The listing builds one solid part. Answer for the finished solid, in the listing's coordinates (mm). A direction names the side the tool comes from. Coordinates: 2 decimals unless noted, no trailing zeros. Loops run counter-clockwise (first coordinate to the right, second up) from the corner with the lowest first, then second, coordinate; pieces in that order, holes last. Notation, with made-up numbers: (38.5, 38.25) - (87.5, 38.25) arc R24 cw to (87.5, 50.25) - close; hole circle Ø6 at (7, 65.25). An arc over 180 degrees is marked (long way). Use one line per item in the form item = value. Start each with the question number.
Autodesk Inventor part; units mm, degrees
ref_plane "YZ Plane" through (0, 0, 0) normal (1, 0, 0) x (0, 1, 0)
ref_plane "XZ Plane" through (0, 0, 0) normal (0, 1, 0) x (-1, 0, 0)
ref_plane "XY Plane" through (0, 0, 0) normal (0, 0, 1) x (1, 0, 0)
sketch "スケッチ1" plane through (0, 0, 0) normal (0, 1, 0) x (-1, 0, 0)
  line L0 (22.5, -27.3) -> (-22.5, -27.3)
  line L1 (-22.5, -27.3) -> (-22.5, 27.3)
  line L2 (-22.5, 27.3) -> (22.5, 27.3)
  line L3 (22.5, 27.3) -> (22.5, -27.3)
  line L4 (22.5, -27.3) -> (-22.5, 27.3) construction
  line L5 (-22.5, -27.3) -> (22.5, 27.3) construction
  point P0 (0, 0)
  dimension "d0" = 45
  dimension "d1" = 54.6
extrude "押し出し1" add sketch "スケッチ1" along normal blind 5
sketch "スケッチ2" plane through (0, 5, 0) normal (0, 1, 0) x (1, 0, 0)
  line L0 (-22.5, 27.3) -> (-22.5, -27.3)
  line L1 (-22.5, -27.3) -> (22.5, -27.3)
  line L2 (22.5, 27.3) -> (-22.5, 27.3)
  point P0 (0, 0)
  point P1 (-12.5, -17.3)
  point P2 (-12.5, 17.3)
  dimension "d4" = 10
  dimension "d5" = 10
  dimension "d6" = 10
hole "穴1" at (-12.5, 5, 17.3) at (-12.5, 5, -17.3) direction (0, -1, 0) diameter 5.5 end through all
sketch "スケッチ3" plane through (0, 5, 0) normal (0, 1, 0) x (1, 0, 0)
  line L0 (-2.5, 20.5) -> (17.5, 20.5)
  line L1 (17.5, 20.5) -> (17.5, -20.5)
  line L2 (17.5, -20.5) -> (-2.5, -20.5)
  line L3 (-2.5, -20.5) -> (-2.5, 20.5)
  line L4 (-2.5, 20.5) -> (17.5, -20.5) construction
  line L5 (17.5, 20.5) -> (-2.5, -20.5) construction
  line L6 (22.5, -27.3) -> (22.5, 27.3)
  circle A0 centre (2.5, -24.3) radius 2
  circle A1 centre (2.5, 24.3) radius 2
  circle A2 centre (12.5, 24.3) radius 2
  circle A3 centre (12.5, -24.3) radius 2
  point P0 (0, 0)
  point P1 (7.5, 0)
  point P2 (7.5, 0)
  dimension "d14" = 5
  dimension "d15" = 41
  dimension "d16" = 20
  dimension "d17" = 24.3
  dimension "d18" = 5
  dimension "d19" = 4
  dimension "d22" = 48.6
  dimension "d29" = 10
extrude "押し出し2" cut sketch "スケッチ3" against normal through all
sketch "スケッチ4" plane through (0, 0, 0) normal (0, -1, 0) x (1, 0, 0)
  line L0 (8.5, -35) -> (6.5, -35)
  line L1 (6.5, -35) -> (6.5, 35)
  line L2 (6.5, 35) -> (8.5, 35)
  line L3 (8.5, 35) -> (8.5, -35)
  line L4 (8.5, -35) -> (6.5, 35) construction
  line L5 (6.5, -35) -> (8.5, 35) construction
  line L6 (17.5, -20.5) -> (-2.5, -20.5)
  point P0 (0, 0)
  point P1 (7.5, 0)
  point P2 (7.5, -20.5)
  point P3 (7.5, 0)
  point P4 (6.5, -20.5)
  point P5 (8.5, -20.5)
  dimension "d36" = 2
  dimension "d37" = 70
extrude "押し出し3" cut sketch "スケッチ4" against normal blind 3
chamfer "面取り1" distance 6 angle 45 4 edges at (22.5, 2.5, -27.3) (22.5, 2.5, 27.3) (-22.5, 2.5, -27.3) (-22.5, 2.5, 27.3)
fillet "フィレット1" radius 1 18 edges at (-22.5, 5, 0) (0, 5, 27.3) (-19.5, 5, 24.3) (19.5, 5, 24.3) (22.5, 5, 0) (19.5, 5, -24.3) (0, 5, -27.3) (-19.5, 5, -24.3) (-22.5, 0, 0) (-19.5, 0, 24.3) (-5, 0, 27.3) (12.5, 0, 27.3) (19.5, 0, 24.3) (22.5, 0, 0) (19.5, 0, -24.3) (12.5, 0, -27.3) (-5, 0, -27.3) (-19.5, 0, -24.3)
equation "\"d22\" = 2 * d17"
equation "\"d29\" = 2 * d18"
properties part number "base1" material "ABS プラスチック"
(1) A cutting plane is placed at B-B (z = -4.5). Determine the outline of the cut face in (x, y).
(2) For faces 1 (the face through (7, 3, 24)), 2 (the face through (19.3, 4.7, -24.1)), 3 (the face through (17.5, 3, 0)), determine the directions among +Z, -Z, +X, -X, +Y, -Y from which every point of the face is accessible in a straight line to the end or side of a thin tool.
(3) A cutting plane is placed at C-C (x = 5.5). Determine the outline of the cut face in (y, z).
(4) A cutting plane is placed at A-A (y = 2.35). Determine the outline of the cut face in (x, z), then the cut area to 3 significant figures.
(5) Find the intervals of material crossed by probe 1 along Z at (x, y) = (-12.5, 1.15); probe 2 along X at (y, z) = (3.25, 17.3); probe 3 along Z at (x, y) = (12.5, 1.75), in increasing order. Write a range as from..to.
(6) Each of these flat-tipped pins is pushed along its axis until it touches: pin 1 Ø8 at (x, z) = (12, -2) entering from -Y; pin 2 Ø1.5 at (y, z) = (1.5, -25.5) entering from +X; pin 3 Ø1.5 at (y, z) = (1, -23) entering from -X; pin 4 Ø0.9 at (y, z) = (1.5, 24.5) entering from +X. Where does it stop, or does it pass through?
(7) A cutting plane is placed at D-D (x = -12.5). Determine the outline of the cut face in (y, z), then the cut area to 3 significant figures.
Evaluation:
q1.outline = (-22.5, 1) arc R1 ccw to (-21.5, 0) - (-2.5, 0) - (-2.5, 5) - (-21.5, 5) arc R1 ccw to (-22.5, 4) - close; (17.5, 0) - (21.5, 0) arc R1 ccw to (22.5, 1) - (22.5, 4) arc R1 ccw to (21.5, 5) - (17.5, 5) - close
q2.face_1 = +Z, -Z, -Y
q2.face_2 = -Z, +X, +Y
q2.face_3 = +Y, -Y
q3.outline = (0, -26.3) arc R1 ccw to (1, -27.3) - (4, -27.3) arc R1 ccw to (5, -26.3) - (5, -20.5) - (0, -20.5) - close; (0, 20.5) - (5, 20.5) - (5, 26.3) arc R1 ccw to (4, 27.3) - (1, 27.3) arc R1 ccw to (0, 26.3) - close
q4.outline = (-22.5, -21.3) - (-16.5, -27.3) - (6.5, -27.3) - (6.5, -20.5) - (-2.5, -20.5) - (-2.5, 20.5) - (6.5, 20.5) - (6.5, 27.3) - (-16.5, 27.3) - (-22.5, 21.3) - close; (8.5, -27.3) - (16.5, -27.3) - (22.5, -21.3) - (22.5, 21.3) - (16.5, 27.3) - (8.5, 27.3) - (8.5, 20.5) - (17.5, 20.5) - (17.5, -20.5) - (8.5, -20.5) - close; hole circle Ø5.5 at (-12.5, -17.3); hole circle Ø5.5 at (-12.5, 17.3); hole circle Ø4 at (2.5, -24.3); hole circle Ø4 at (2.5, 24.3); hole circle Ø4 at (12.5, -24.3); hole circle Ø4 at (12.5, 24.3)
q4.area = 1,440 mm^2
q5.probe_1 = -27.3..-20.05, -14.55..14.55, 20.05..27.3
q5.probe_2 = -22.5..-15.25, -9.75..-2.5, 17.5..22.5
q5.probe_3 = -27.3..-26.3, -22.3..-20.5, 20.5..22.3, 26.3..27.3
q6.pin_1 = through
q6.pin_2 = 19.05
q6.pin_3 = -21.55
q6.pin_4 = 19.75
q7.outline = (0, -26.3) arc R1 ccw to (1, -27.3) - (4, -27.3) arc R1 ccw to (5, -26.3) - (5, -20.05) - (0, -20.05) - close; (0, -14.55) - (5, -14.55) - (5, 14.55) - (0, 14.55) - close; (0, 20.05) - (5, 20.05) - (5, 26.3) arc R1 ccw to (4, 27.3) - (1, 27.3) arc R1 ccw to (0, 26.3) - close
q7.area = 217 mm^2
